```python
from build123d import *

# Parameters (mm, degrees)
F1_DEPTH = 5


with BuildPart() as f1:
    # F0 (on Top) → F1 (new body)
    with BuildSketch(Plane.XY):
        with BuildLine():
            ThreePointArc((-24.457556, 78.779693), (-28.980906, 79.883488), (-27.460124, 84.284202))
            ThreePointArc((-27.460124, 84.284202), (-27.025335, 84.591656), (-26.889149, 85.106458))
            ThreePointArc((-26.889149, 85.106458), (-27.416891, 85.177568), (-27.867286, 84.893467))
            ThreePointArc((-27.867286, 84.893467), (-32.515034, 85.171848), (-31.804469, 89.773387))
            ThreePointArc((-31.804469, 89.773387), (-31.431566, 90.153534), (-31.38949, 90.684381))
            ThreePointArc((-31.38949, 90.684381), (-31.921448, 90.660115), (-32.313877, 90.300159))
            ThreePointArc((-32.313877, 90.300159), (-36.936641, 89.744179), (-37.059131, 94.398646))
            ThreePointArc((-37.059131, 94.398646), (-36.760099, 94.839268), (-36.813485, 95.369096))
            ThreePointArc((-36.813485, 95.369096), (-37.332562, 95.250236), (-37.654411, 94.825994))
            ThreePointArc((-37.654411, 94.825994), (-42.103612, 93.453522), (-43.055221, 98.011318))
            ThreePointArc((-43.055221, 98.011318), (-42.83967, 98.498254), (-42.986803, 99.010035))
            ThreePointArc((-42.986803, 99.010035), (-43.476314, 98.800401), (-43.71724, 98.325508))
            ThreePointArc((-43.71724, 98.325508), (-47.849876, 96.180657), (-49.600018, 100.495291))
            ThreePointArc((-49.600018, 100.495291), (-49.474877, 101.012889), (-49.711027, 101.490174))
            ThreePointArc((-49.711027, 101.490174), (-50.155241, 101.196503), (-50.307499, 100.686223))
            ThreePointArc((-50.307499, 100.686223), (-53.990744, 97.83793), (-56.483168, 101.770726))
            ThreePointArc((-56.483168, 101.770726), (-56.452459, 102.302351), (-56.770037, 102.7298))
            ThreePointArc((-56.770037, 102.7298), (-57.154674, 102.36153), (-57.213372, 101.832264))
            ThreePointArc((-57.213372, 101.832264), (-60.328843, 98.372076), (-63.483441, 101.79663))
            ThreePointArc((-63.483441, 101.79663), (-63.54815, 102.325195), (-63.936949, 102.689069))
            ThreePointArc((-63.936949, 102.689069), (-64.249648, 102.258038), (-64.212898, 101.726797))
            ThreePointArc((-64.212898, 101.726797), (-66.660462, 97.765926), (-70.375842, 100.572172))
            ThreePointArc((-70.375842, 100.572172), (-70.53389, 101.080688), (-70.981413, 101.369292))
            ThreePointArc((-70.981413, 101.369292), (-71.212123, 100.889353), (-71.081107, 100.37321))
            ThreePointArc((-71.081107, 100.37321), (-72.782097, 96.038964), (-76.938844, 98.136705))
            ThreePointArc((-76.938844, 98.136705), (-77.185151, 98.608829), (-77.677014, 98.812886))
            ThreePointArc((-77.677014, 98.812886), (-77.818321, 98.299465), (-77.597249, 97.815011))
            ThreePointArc((-77.597249, 97.815011), (-78.496993, 93.246694), (-82.961506, 94.568508))
            ThreePointArc((-82.961506, 94.568508), (-83.288156, 94.989064), (-83.80855, 95.102017))
            ThreePointArc((-83.80855, 95.102017), (-83.855911, 94.571616), (-83.55189, 94.134421))
            ThreePointArc((-83.55189, 94.134421), (-83.62147, 89.478863), (-88.250255, 89.982265))
            ThreePointArc((-88.250255, 89.982265), (-88.646749, 90.337737), (-89.178949, 90.355955))
            ThreePointArc((-89.178949, 90.355955), (-89.130842, 89.825621), (-88.753642, 89.449737))
            ThreePointArc((-88.753642, 89.449737), (-87.990823, 84.856572), (-92.635107, 84.525383))
            ThreePointArc((-92.635107, 84.525383), (-93.088701, 84.804346), (-93.615601, 84.727242))
            ThreePointArc((-93.615601, 84.727242), (-93.473573, 84.214021), (-93.035318, 83.911529))
            ThreePointArc((-93.035318, 83.911529), (-91.464616, 79.528385), (-95.975128, 78.373249))
            ThreePointArc((-95.975128, 78.373249), (-96.471244, 78.566737), (-96.975909, 78.396791))
            ThreePointArc((-96.975909, 78.396791), (-96.744524, 77.917177), (-96.2593, 77.6978))
            ThreePointArc((-96.2593, 77.6978), (-93.931199, 73.665554), (-98.162968, 71.723599))
            ThreePointArc((-98.162968, 71.723599), (-98.68566, 71.825392), (-99.15187, 71.568066))
            ThreePointArc((-99.15187, 71.568066), (-98.838564, 71.137476), (-98.321967, 71.008264))
            ThreePointArc((-98.321967, 71.008264), (-95.311294, 67.456516), (-99.128308, 64.790157))
            ThreePointArc((-99.128308, 64.790157), (-99.660775, 64.796985), (-100.073546, 64.460549))
            ThreePointArc((-100.073546, 64.460549), (-99.68839, 64.092821), (-99.157023, 64.057928))
            ThreePointArc((-99.157023, 64.057928), (-95.560544, 61.100835), (-98.84012, 57.795771))
            ThreePointArc((-98.84012, 57.795771), (-99.36525, 57.707413), (-99.711314, 57.302681))
            ThreePointArc((-99.711314, 57.302681), (-99.266688, 57.009635), (-98.73763, 57.070181))
            ThreePointArc((-98.73763, 57.070181), (-94.670938, 54.802786), (-97.307668, 50.965246))
            ThreePointArc((-97.307668, 50.965246), (-97.808582, 50.784542), (-98.076817, 50.324522))
            ThreePointArc((-98.076817, 50.324522), (-97.58701, 50.115576), (-97.077265, 50.269617))
            ThreePointArc((-97.077265, 50.269617), (-92.671068, 48.764795), (-94.580205, 44.518119))
            ThreePointArc((-94.580205, 44.518119), (-95.040803, 44.250878), (-95.222588, 43.750355))
            ThreePointArc((-95.222588, 43.750355), (-94.703344, 43.632226), (-94.229296, 43.874809))
            ThreePointArc((-94.229296, 43.874809), (-89.625212, 43.180928), (-90.745395, 38.661608))
            ThreePointArc((-90.745395, 38.661608), (-91.150874, 38.316418), (-91.240365, 37.79148))
            ThreePointArc((-91.240365, 37.79148), (-90.708373, 37.767964), (-90.285258, 38.091294))
            ThreePointArc((-90.285258, 38.091294), (-85.631266, 38.230654), (-85.926492, 33.583945))
            ThreePointArc((-85.926492, 33.583945), (-86.263818, 33.171902), (-86.25814, 32.639421))
            ThreePointArc((-86.25814, 32.639421), (-85.730498, 32.711273), (-85.371916, 33.104957))
            ThreePointArc((-85.371916, 33.104957), (-80.817599, 34.07308), (-80.278379, 29.448331))
            ThreePointArc((-80.278379, 29.448331), (-80.53671, 28.982677), (-80.436046, 28.459767))
            ThreePointArc((-80.436046, 28.459767), (-79.929713, 28.624679), (-79.647188, 29.076063))
            ThreePointArc((-79.647188, 29.076063), (-75.338926, 30.841833), (-73.98259, 26.387687))
            ThreePointArc((-73.98259, 26.387687), (-74.153625, 25.88339), (-73.961209, 25.386858))
            ThreePointArc((-73.961209, 25.386858), (-73.492459, 25.639528), (-73.295072, 26.134105))
            ThreePointArc((-73.295072, 26.134105), (-69.371337, 28.640768), (-67.241479, 24.500386))
            ThreePointArc((-67.241479, 24.500386), (-67.319719, 23.973653), (-67.041736, 23.519458))
            ThreePointArc((-67.041736, 23.519458), (-66.625635, 23.851766), (-66.519731, 24.37364))
            ThreePointArc((-66.519731, 24.37364), (-63.106633, 27.54063), (-60.271709, 23.847086))
            ThreePointArc((-60.271709, 23.847086), (-60.254641, 23.314848), (-59.900025, 22.917587))
            ThreePointArc((-59.900025, 22.917587), (-59.549947, 23.318853), (-59.538929, 23.85125))
            ThreePointArc((-59.538929, 23.85125), (-56.746169, 27.576777), (-53.297296, 24.448785))
            ThreePointArc((-53.297296, 24.448785), (-53.185466, 23.928148), (-52.765616, 23.600591))
            ThreePointArc((-52.765616, 23.600591), (-52.492813, 24.057917), (-52.577035, 24.583726))
            ThreePointArc((-52.577035, 24.583726), (-50.494374, 28.748049), (-46.542401, 26.286145))
            ThreePointArc((-46.542401, 26.286145), (-46.339406, 25.793842), (-45.867814, 25.546516))
            ThreePointArc((-45.867814, 25.546516), (-45.681054, 26.045204), (-45.857809, 26.547524))
            ThreePointArc((-45.857809, 26.547524), (-44.552187, 31.016798), (-40.224134, 29.30011))
            ThreePointArc((-40.224134, 29.30011), (-39.936496, 28.851966), (-39.428322, 28.69282))
            ThreePointArc((-39.428322, 28.69282), (-39.333607, 29.21684), (-39.597215, 29.679528))
            ThreePointArc((-39.597215, 29.679528), (-39.110594, 34.310107), (-34.545568, 33.39381))
            ThreePointArc((-34.545568, 33.39381), (-34.182534, 33.004227), (-33.654109, 32.938377))
            ThreePointArc((-33.654109, 32.938377), (-33.654484, 33.470888), (-33.996471, 33.879071))
            ThreePointArc((-33.996471, 33.879071), (-34.344492, 38.522124), (-29.689217, 38.435669))
            ThreePointArc((-29.689217, 38.435669), (-29.262454, 38.117169), (-28.730764, 38.146731))
            ThreePointArc((-28.730764, 38.146731), (-28.826216, 38.670618), (-29.235592, 39.011177))
            ThreePointArc((-29.235592, 39.011177), (-30.407069, 43.517473), (-25.811168, 44.263639))
            ThreePointArc((-25.811168, 44.263639), (-25.334394, 44.026459), (-24.816526, 44.150483))
            ThreePointArc((-24.816526, 44.150483), (-25.003988, 44.648907), (-25.467594, 44.910896))
            ThreePointArc((-25.467594, 44.910896), (-27.424875, 49.135598), (-23.036066, 50.690403))
            ThreePointArc((-23.036066, 50.690403), (-22.524603, 50.542166), (-22.037204, 50.756665))
            ThreePointArc((-22.037204, 50.756665), (-22.31065, 51.213607), (-22.813585, 51.388606))
            ThreePointArc((-22.813585, 51.388606), (-25.493762, 55.19593), (-21.453104, 57.5094))
            ThreePointArc((-21.453104, 57.5094), (-20.923392, 57.45487), (-20.482125, 57.752951))
            ThreePointArc((-20.482125, 57.752951), (-20.832767, 58.153724), (-21.358867, 58.236108))
            ThreePointArc((-21.358867, 58.236108), (-24.675796, 61.503683), (-21.113159, 64.501462))
            ThreePointArc((-21.113159, 64.501462), (-20.582223, 64.542392), (-20.201272, 64.914474))
            ThreePointArc((-20.201272, 64.914474), (-20.61784, 65.246197), (-21.150196, 65.233318))
            ThreePointArc((-21.150196, 65.233318), (-24.997268, 67.856121), (-22.027159, 71.441858))
            ThreePointArc((-22.027159, 71.441858), (-21.512063, 71.576933), (-21.203672, 72.011056))
            ThreePointArc((-21.203672, 72.011056), (-21.672777, 72.263067), (-22.194278, 72.155339))
            ThreePointArc((-22.194278, 72.155339), (-26.447846, 74.049071), (-24.165725, 78.107518))
            ThreePointArc((-24.165725, 78.107518), (-23.683026, 78.332396), (-23.457107, 78.814608))
            ThreePointArc((-23.457107, 78.814608), (-23.963671, 78.978807), (-24.457556, 78.779693))
        make_face()
    extrude(amount=F1_DEPTH)


solid = f1.part
```
Source: CAD feature listing. Evaluate the final solid. Frame: model axes, mm. Coordinates: 2 decimals unless noted, no trailing zeros. Write each loop counter-clockwise with the first axis right and the second up, starting at its lowest first coordinate (ties: lowest second). Pieces come first, ordered by that corner, then holes. Notation, with made-up numbers: (28, 48) - (87, 48) arc R17 cw to (87, 78) - close; hole circle Ø9 at (64.25, 46.5). An arc over 180 degrees is marked (long way). Answer as a JSON object with one key per item and string values.
Q1. Section query A-A, the plane y = 74. Output: boundary loops of the cut face in (x, z), plus the area to 3 significant figures.
Ans:
{"outline": "(-93.84, 0) - (-26.43, 0) - (-26.43, 5) - (-93.84, 5) - close", "area": "337 mm2"}
Q2. Section query B-B, the plane y = 82.5. Output: boundary loops of the cut face in (x, z).
Ans:
{"outline": "(-91.47, 0) - (-29.16, 0) - (-29.16, 5) - (-91.47, 5) - close"}
Q3. Draft query along X for faces 1 (the cylindrical face through (-63.18, 27.546, 2.465)), 2 (the flat face through (-61, 63, 5)). Return one class per face: released by +X, released by -X, zero draft, split by the parting line, or undercut.
Ans:
{"face 1": "undercut", "face 2": "zero draft"}
Q4. Material intervals for line 1 (X direction, y = 33, z = 4); line 2 (X direction, y = 68, z = 1.55); line 3 (Y direction, x = -24, z = 0.7), sorted ascending. Write a range as [from, to].
Ans:
{"line 1": "x = [-86.3, -85.42], [-79.88, -40.15], [-34.17, -33.63]", "line 2": "x = [-95.29, -25.01]", "line 3": "y = [51.02, 51.79], [57.24, 59.43], [63.33, 65.97], [70.62, 71.94], [78.14, 78.98]"}
Q5. First-contact query: pin 1 Ø3 at (y, z) = (75, 3.5) entering from +X; pin 2 Ø8 at (x, y) = (-26.22, 81.39) entering from +Z; pin 3 Ø4 at (x, y) = (-43.17, 28.19) entering from -Z; pin 4 Ø2 at (x, z) = (-81, 3) entering from +Y. Flat tips, straight axial feed; report the tip coordinate or a pass-through.
Ans:
{"pin 1": "stops at x = -26.21", "pin 2": "stops at z = 5", "pin 3": "passes through", "pin 4": "stops at y = 93.41"}
